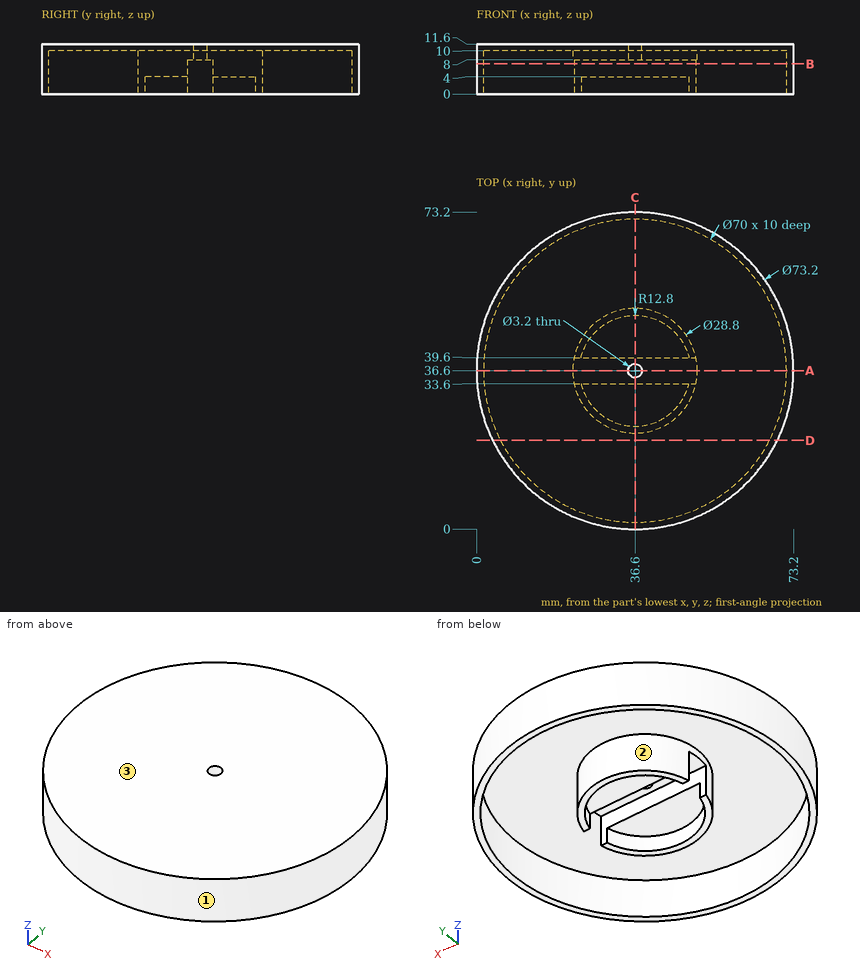
Design review of the part shown in the three views and the two pictorial views. Dimensions are in mm from the part's minimum x, y and z. Round coordinates to 2 decimals unless told otherwise and drop trailing zeros. Loops run counter-clockwise (first coordinate to the right, second up) from the corner with the lowest first, then second, coordinate; pieces in that order, holes last. Notation, with made-up numbers: (78.5, 64) - (91.5, 64) arc R11 cw to (91.5, 75) - close; hole circle Ø2 at (17, 10.25). An arc over 180 degrees is marked (long way). Use CSV: the item, a comma, the result in double quotes.
(1) Clearance check with flat-ended pins moving along their axes: P1, Ø3, axis at x = 35.5, y = 37.5, coming from the -Z side; P2, Ø1.5, axis at x = 17, z = 9, coming from the -Y side; P3, Ø1.5, axis at x = 59.5, z = 10, coming from the +Y side. State where each tip first meets the part, or that it passes through.
Working result:
P1,"stops at z = 8"
P2,"stops at y = 5.23"
P3,"stops at y = 65.74"
(2) The part is to be moulded in two halves that separate along Y. For the marked faces 1, 2 and 3, say which applies: pulls with the +Y half, pulls with the -Y half, needs draft (parallel to the pull), parting line crosses it, or undercut.
Working result:
face 1,"parting line crosses it"
face 2,"undercut"
face 3,"needs draft"
(3) For line 1 (Y direction, x = 36.6, z = 7); line 2 (Y direction, x = 36.6, z = 9.65); line 3 (Z direction, x = 52.5, y = 40), list the stretches that pass through material, from the lowest coordinate up.
Working result:
line 1,"y = 0 to 1.6, 22.2 to 33.6, 39.6 to 51, 71.6 to 73.2"
line 2,"y = 0 to 1.6, 22.2 to 35, 38.2 to 51, 71.6 to 73.2"
line 3,"z = 10 to 11.6"
(4) Take a section at A-A, the plane y = 36.6. Give the boundary of the cut face in (x, z).
Working result:
outline,"(0, 0) - (1.6, 0) - (1.6, 10) - (22.2, 10) - (22.2, 8) - (35, 8) - (35, 11.6) - (0, 11.6) - close; (38.2, 8) - (51, 8) - (51, 10) - (71.6, 10) - (71.6, 0) - (73.2, 0) - (73.2, 11.6) - (38.2, 11.6) - close"
(5) Take a section at D-D, the plane y = 20.5. Give the boundary of the cut face in (x, z), plus the area to 3 significant figures.
Working result:
outline,"(3.73, 0) - (5.52, 0) - (5.52, 10) - (67.68, 10) - (67.68, 0) - (69.47, 0) - (69.47, 11.6) - (3.73, 11.6) - close"
area,"141 mm^2"
(6) Take a section at B-B, the plane z = 7. Give the boundary of the cut face in (x, y), plus the area to 3 significant figures.
Working result:
outline,"circle Ø73.2 at (36.6, 36.6); (22.52, 33.6) arc R14.4 ccw to (50.68, 33.6) - close; (22.52, 39.6) - (50.68, 39.6) arc R14.4 ccw to start; hole circle Ø70 at (36.6, 36.6)"
area,"840 mm^2"
(7) Take a section at C-C, the plane x = 36.6. Give the boundary of the cut face in (y, z), plus the area to 3 significant figures.
Working result:
outline,"(0, 0) - (1.6, 0) - (1.6, 10) - (22.2, 10) - (22.2, 0) - (23.8, 0) - (23.8, 4) - (33.6, 4) - (33.6, 8) - (35, 8) - (35, 11.6) - (0, 11.6) - close; (38.2, 8) - (39.6, 8) - (39.6, 4) - (49.4, 4) - (49.4, 0) - (51, 0) - (51, 10) - (71.6, 10) - (71.6, 0) - (73.2, 0) - (73.2, 11.6) - (38.2, 11.6) - close"
area,"299 mm^2"
